Could you check a few things on this model? Use its own coordinates, in mm. A direction names the side the tool comes from. Round coordinates to 2 decimals unless told otherwise and drop trailing zeros. Write each loop counter-clockwise with the first axis right and the second up, starting at its lowest first coordinate (ties: lowest second). Pieces come first, ordered by that corner, then holes. Notation, with made-up numbers: (-6.75, 34) - (29.25, 34) arc R13 cw to (29.25, 50) - close; hole circle Ø3 at (37.5, 63). An arc over 180 degrees is marked (long way). Put each result on its own line as item: value.
from build123d import *

# Parameters (mm, degrees)
F1_DEPTH = 3.175
F3_D     = 5.08
F5_DEPTH = 3.176


with BuildPart() as f1:
    # F0 (on Top) → F1 (new body)
    with BuildSketch(Plane.XY):
        with BuildLine():
            ThreePointArc((73.025, 47.625), (71.165128, 52.115128), (66.675, 53.975))
            Line((66.675, 53.975), (-66.675, 53.975))
            ThreePointArc((-66.675, 53.975), (-71.165128, 52.115128), (-73.025, 47.625))
            Line((-73.025, 47.625), (-73.025, -47.625))
            ThreePointArc((-73.025, -47.625), (-71.165128, -52.115128), (-66.675, -53.975))
            Line((-66.675, -53.975), (66.675, -53.975))
            ThreePointArc((66.675, -53.975), (71.165128, -52.115128), (73.025, -47.625))
            Line((73.025, -47.625), (73.025, 47.625))
        make_face()
    extrude(amount=F1_DEPTH)

    # F3 (through all)
    with Locations(Plane.XY.offset(3.175)):
        with Locations((-66.675, 47.625), (66.675, 47.625), (66.675, -47.625), (-66.675, -47.625)):
            Hole(F3_D / 2)

    # F4 (on face) → F5 (cut, through all)
    with BuildSketch(Plane.XY.offset(3.175)):
        with BuildLine():
            Line((-32.811304, -8.775606), (-11.638696, -8.775606))
            ThreePointArc((-11.638696, -8.775606), (-9.393632, -7.845671), (-8.463696, -5.600606))
            Line((-8.463696, -5.600606), (-8.463696, 11.950606))
            ThreePointArc((-8.463696, 11.950606), (-9.393632, 14.195671), (-11.638696, 15.125606))
            Line((-11.638696, 15.125606), (-32.811304, 15.125606))
            ThreePointArc((-32.811304, 15.125606), (-35.056368, 14.195671), (-35.986304, 11.950606))
            Line((-35.986304, 11.950606), (-35.986304, -5.600606))
            ThreePointArc((-35.986304, -5.600606), (-35.056368, -7.845671), (-32.811304, -8.775606))
        make_face()
    extrude(amount=-F5_DEPTH, mode=Mode.SUBTRACT)


solid = f1.part
(1) Imagine slicing it at B-B, the plane x = -34.5. List the corners of the cut face in (y, z) for me (3 decimals), then the cut area to 3 significant figures.
Values found:
outline: (-53.975, 0) - (-8.289, 0) - (-8.289, 3.175) - (-53.975, 3.175) - close; (14.639, 0) - (53.975, 0) - (53.975, 3.175) - (14.639, 3.175) - close
area: 270 mm^2
(2) For faces 1 (the face through (-1, -53.975, 2)), 2 (the face through (-35.986, 3, 2)), which set-ups out of +Z, -Z, +X, -X, +Y, -Y let a thin tool reach every point of the face, with its end or its side?
Values found:
face 1: +Z, -Z, +X, -X, -Y
face 2: +Z, -Z
(3) If we mould it in two halves opening along Y, with no side actions, what happens to faces 3 (the face through (-73.025, 1, 2)), 4 (the face through (-22, -8.776, 2)), 5 (the face through (-71.12, 52.16, 1.57)), 6 (the face through (71.12, -52.16, 1.57))? For each: pulls with the +Y half, pulls with the -Y half, needs draft (parallel to the pull), parting line crosses it, or undercut.
Values found:
face 3: needs draft
face 4: undercut
face 5: pulls with the +Y half
face 6: pulls with the -Y half
(4) Imagine slicing it at A-A, the plane z = 2.35. List the corners of the cut face in (x, y) for me (3 decimals), then the cut area to 3 significant figures.
Values found:
outline: (-73.025, -47.625) arc R6.35 ccw to (-66.675, -53.975) - (66.675, -53.975) arc R6.35 ccw to (73.025, -47.625) - (73.025, 47.625) arc R6.35 ccw to (66.675, 53.975) - (-66.675, 53.975) arc R6.35 ccw to (-73.025, 47.625) - close; hole circle Ø5.08 at (-66.675, -47.625); hole circle Ø5.08 at (-66.675, 47.625); hole (-35.986, -5.601) arc R3.175 ccw to (-32.811, -8.776) - (-11.639, -8.776) arc R3.175 ccw to (-8.464, -5.601) - (-8.464, 11.951) arc R3.175 ccw to (-11.639, 15.126) - (-32.811, 15.126) arc R3.175 ccw to (-35.986, 11.951) - close; hole circle Ø5.08 at (66.675, -47.625); hole circle Ø5.08 at (66.675, 47.625)
area: 15,000 mm^2
(5) Please list where these lines run through material, in increasing order: probe 1 along X at (y, z) = (-3.5, 0.35) (3 decimals); probe 2 along Y at (x, z) = (-16, 2.65) (3 decimals); probe 3 along X at (y, z) = (49, 0.55). Write a range as from..to.
Values found:
probe 1: x = -73.025..-35.986, -8.464..73.025
probe 2: y = -53.975..-8.776, 15.126..53.975
probe 3: x = -72.87..-68.81, -64.54..64.54, 68.81..72.87
